Read the model definition and answer for the solid it produces. Units are mm, in the model's axes. A direction names the side the tool comes from. Coordinates: 2 decimals unless noted, no trailing zeros. Write each loop counter-clockwise with the first axis right and the second up, starting at its lowest first coordinate (ties: lowest second). Pieces come first, ordered by that corner, then holes.
1) The part is cut by section A-A (y = 23.5). Determine the outline of the cut face in (x, z), then the cut area to 3 significant figures.
2) Which of the six approach directions +Z, -Z, +X, -X, +Y, -Y give full straight-line access (tool end or side, diameter ignored) to faces 1 (the face through (84, 5, -2)), 2 (the face through (44, 17, 1)), 3 (the face through (64, 9.5, -70)), 4 (the face through (25.29, 5.19, -69.73)), 5 (the face through (44, 17, -94))?
3) The part is cut by section C-C (z = -78). Determine the outline of the cut face in (x, y).
4) The part is cut by section B-B (x = 14.85). Determine the outline of the cut face in (y, z).
5) Determine the mould class of faces 6 (the face through (73.06, 5.19, -87.65)), 7 (the face through (86, 5, -4)), 8 (the face through (44.126, 34.03, -91.986)) for opening direction X: +X half, -X half, draft (parallel to the pull), parting line (faces both ways), or undercut.
6) The part is cut by section D-D (x = 45). Determine the outline of the cut face in (y, z), then the cut area to 3 significant figures.
7) Each of these flat-tipped pins is pushed along its axis until it touches: pin 1 Ø0.6 at (x, y) = (85.5, 7) entering from -Z; pin 2 Ø3.5 at (x, z) = (5, -69) entering from +Y; pin 3 Ø2 at (y, z) = (4, -4) entering from -X. Where does it stop, or does it pass through?
8) Find the intervals of material crossed by line 1 (Z direction, x = 14.85, y = 0.4); line 2 (Z direction, x = 45, y = 19); line 3 (Y direction, x = 76, z = -38), in increasing order.
Autodesk Inventor part; units mm, degrees
ref_plane "YZ Plane" through (0, 0, 0) normal (1, 0, 0) x (0, 1, 0)
ref_plane "XZ Plane" through (0, 0, 0) normal (0, 1, 0) x (-1, 0, 0)
ref_plane "XY Plane" through (0, 0, 0) normal (0, 0, 1) x (1, 0, 0)
sketch "Sketch1" plane through (0, 0, 0) normal (0, 1, 0) x (-1, 0, 0)
  line L0 (0, 0) -> (-88, 0)
  line L1 (-88, 0) -> (-88, -94)
  line L2 (-88, -94) -> (0, -94)
  line L3 (0, -94) -> (0, 0)
  line L4 (0, -94) -> (0, -75.65)
  line L5 (0, -94) -> (-14.85, -94)
  circle A0 centre (-14.85, -75.65) radius 8.5
  line L6 (-44, -88.9444) -> (-44, -54.2543) construction
  circle A1 centre (-73.15, -75.65) radius 8.5
  dimension "d0" = 88
  dimension "d1" = 94
  dimension "d2" = 18.35
  dimension "d3" = 14.85
  dimension "d4" = 17
extrude "Extrusion1" add sketch "Sketch1" along normal blind 1
sketch "Sketch2" plane through (0, 1, 0) normal (0, 1, 0) x (1, 0, 0)
  line L0 (88, 94) -> (0, 94) construction
  line L1 (0, 94) -> (0, 0) construction
  line L2 (0, 0) -> (88, 0) construction
  line L3 (88, 0) -> (88, 94) construction
  circle A0 centre (73.15, 75.65) radius 8.5 construction
  circle A1 centre (14.85, 75.65) radius 8.5 construction
  line L4 (0, 94) -> (88, 94) construction
  line L5 (88, 94) -> (88, 95) construction
  line L6 (88, 95) -> (0, 95) construction
  line L7 (0, 95) -> (0, 94) construction
  line L8 (0, 0) -> (88, 0) construction
  line L9 (88, 0) -> (88, -1) construction
  line L10 (88, -1) -> (0, -1) construction
  line L11 (0, -1) -> (0, 0) construction
  line L12 (88, 95) -> (0, 95)
  line L13 (0, 95) -> (0, 94)
  line L14 (0, 94) -> (88, 94)
  line L15 (88, 94) -> (88, 95)
  line L16 (0, 0) -> (88, 0)
  line L17 (88, 0) -> (88, -1)
  line L18 (88, -1) -> (0, -1)
  line L19 (0, -1) -> (0, 0)
  dimension "d7" = 1
  dimension "d8" = 1
extrude "Extrusion2" add sketch "Sketch2" against normal blind 1
sketch "Sketch3" plane through (0, 1, 0) normal (0, 1, 0) x (1, 0, 0)
  line L0 (0, 95) -> (0, -1) construction
  line L1 (0, -1) -> (88, -1) construction
  line L2 (88, -1) -> (88, 95) construction
  line L3 (88, 95) -> (0, 95) construction
  circle A0 centre (73.15, 75.65) radius 8.5 construction
  circle A1 centre (14.85, 75.65) radius 8.5 construction
  line L4 (0, 0) -> (4, 0) construction
  line L5 (4, 0) -> (4, 4) construction
  line L6 (4, 4) -> (0, 4) construction
  line L7 (0, 4) -> (0, 0) construction
  line L8 (88, 0) -> (84, 0) construction
  line L9 (84, 0) -> (84, 4) construction
  line L10 (84, 4) -> (88, 4) construction
  line L11 (88, 4) -> (88, 0) construction
  line L12 (4, 4) -> (2, 4) construction
  line L13 (2, 4) -> (2, 2) construction
  line L14 (2, 2) -> (4, 2) construction
  line L15 (4, 2) -> (4, 4) construction
  line L16 (2, 2) -> (6, 2)
  line L17 (6, 2) -> (6, 4)
  line L18 (6, 4) -> (2, 4)
  line L19 (2, 4) -> (2, 2)
  line L20 (2, 2) -> (4, 2)
  line L21 (4, 2) -> (4, 6)
  line L22 (4, 6) -> (2, 6)
  line L23 (2, 6) -> (2, 2)
  line L24 (86, 2) -> (82, 2)
  line L25 (82, 2) -> (82, 4)
  line L26 (82, 4) -> (86, 4)
  line L27 (86, 4) -> (86, 2)
  line L28 (86, 2) -> (84, 2)
  line L29 (84, 2) -> (84, 6)
  line L30 (84, 6) -> (86, 6)
  line L31 (86, 6) -> (86, 2)
  line L32 (44, 4.3599) -> (37, 4.3599) construction
  line L33 (88, -1) -> (0, -1) construction
  line L34 (37, -1) -> (51, -1) construction
  line L35 (51, -1) -> (51, 0) construction
  line L36 (51, 0) -> (37, 0) construction
  line L37 (37, 0) -> (37, -1) construction
  line L38 (37, -1) -> (51, -1)
  line L39 (51, -1) -> (51, 0)
  line L40 (51, 0) -> (37, 0)
  line L41 (37, 0) -> (37, -1)
  line L42 (0, 95) -> (88, 95)
  line L43 (37, 95) -> (51, 95)
  line L44 (51, 95) -> (51, 94)
  line L45 (51, 94) -> (37, 94)
  line L46 (37, 94) -> (37, 95)
  circle A2 centre (14.85, 75.65) radius 10.5
  circle A3 centre (14.85, 75.65) radius 12
  line L47 (14.85, 75.65) -> (26.85, 75.65) construction
  line L48 (14.85, 75.65) -> (20.85, 86.0423) construction
  line L49 (14.85, 75.65) -> (8.85, 86.0423) construction
  line L50 (14.85, 75.65) -> (2.85, 75.65) construction
  line L51 (14.85, 75.65) -> (8.85, 65.2577) construction
  line L52 (14.85, 75.65) -> (20.85, 65.2577) construction
  line L53 (9.6, 84.7433) -> (8.85, 86.0423) construction
  line L54 (9.6, 84.7433) -> (8.85, 86.0423)
  line L55 (20.85, 86.0423) -> (20.1, 84.7433)
  line L56 (25.35, 75.65) -> (26.85, 75.65)
  line L57 (20.85, 65.2577) -> (20.1, 66.5567)
  line L58 (9.6, 66.5567) -> (8.85, 65.2577)
  line L59 (4.35, 75.65) -> (2.85, 75.65)
  line L60 (44, 84.7433) -> (44, 74.6259) construction
  circle A4 centre (73.15, 75.65) radius 8.5 construction
  circle A5 centre (73.15, 75.65) radius 10.5
  circle A6 centre (73.15, 75.65) radius 12
  line L61 (73.15, 75.65) -> (61.15, 75.65) construction
  line L62 (73.15, 75.65) -> (67.15, 86.0423) construction
  line L63 (73.15, 75.65) -> (79.15, 86.0423) construction
  line L64 (73.15, 75.65) -> (85.15, 75.65) construction
  line L65 (73.15, 75.65) -> (79.15, 65.2577) construction
  line L66 (73.15, 75.65) -> (67.15, 65.2577) construction
  line L67 (78.4, 84.7433) -> (79.15, 86.0423) construction
  line L68 (78.4, 84.7433) -> (79.15, 86.0423)
  line L69 (67.15, 86.0423) -> (67.9, 84.7433)
  line L70 (62.65, 75.65) -> (61.15, 75.65)
  line L71 (67.15, 65.2577) -> (67.9, 66.5567)
  line L72 (78.4, 66.5567) -> (79.15, 65.2577)
  line L73 (83.65, 75.65) -> (85.15, 75.65)
  point P0 (84, 4)
  dimension "d11" = 4
  dimension "d12" = 4
  dimension "d13" = 4
  dimension "d14" = 4
  dimension "d15" = 2
  dimension "d16" = 2
  dimension "d17" = 4
  dimension "d18" = 4
  dimension "d19" = 4
  dimension "d20" = 2
  dimension "d21" = 4
  dimension "d22" = 7
  dimension "d23" = 14
  dimension "d24" = 14
  dimension "d25" = 1
  dimension "d26" = 2
  dimension "d27" = 1.5
  dimension "d30" = 360
extrude "Extrusion3" add sketch "Sketch3" along normal blind 8.5 contours L19 L18 L21 L16 | L21 L18 L17 L16 | L23 L22 L21 L18 | L24 L29 L26 L27 | L24 L25 L26 L29 | L26 L29 L30 L31 | L56 A3 L57 A2 | A2 L54 A3 L55 | L58 A3 L59 A2 | L73 A6 L72 A5 | A5 L69 A6 L68 | L71 A6 L70 A5
sketch "Sketch4" plane through (0, 1, 0) normal (0, 1, 0) x (1, 0, 0)
  line L0 (2.85, 75.65) -> (4.35, 75.65) construction
  arc A0 (4.35, 75.65) -> (9.6, 66.5567) centre (14.85, 75.65) ccw construction
  line L1 (9.6, 66.5567) -> (8.85, 65.2577) construction
  arc A1 (2.85, 75.65) -> (8.85, 65.2577) centre (14.85, 75.65) ccw construction
  line L2 (84, 6) -> (86, 6) construction
  line L3 (86, 6) -> (86, 2) construction
  line L4 (86, 2) -> (82, 2) construction
  line L5 (82, 2) -> (82, 4) construction
  line L6 (82, 4) -> (84, 4) construction
  line L7 (84, 4) -> (84, 6) construction
  arc A2 (62.65, 75.65) -> (67.9, 66.5567) centre (73.15, 75.65) ccw construction
  line L8 (67.9, 66.5567) -> (67.15, 65.2577) construction
  arc A3 (61.15, 75.65) -> (67.15, 65.2577) centre (73.15, 75.65) ccw construction
  line L9 (61.15, 75.65) -> (62.65, 75.65) construction
  line L10 (25.35, 75.65) -> (26.85, 75.65) construction
  arc A4 (20.85, 65.2577) -> (26.85, 75.65) centre (14.85, 75.65) ccw construction
  line L11 (20.85, 65.2577) -> (20.1, 66.5567) construction
  arc A5 (20.1, 66.5567) -> (25.35, 75.65) centre (14.85, 75.65) ccw construction
  arc A6 (78.4, 84.7433) -> (67.9, 84.7433) centre (73.15, 75.65) ccw construction
  line L12 (67.9, 84.7433) -> (67.15, 86.0423) construction
  arc A7 (79.15, 86.0423) -> (67.15, 86.0423) centre (73.15, 75.65) ccw construction
  line L13 (79.15, 86.0423) -> (78.4, 84.7433) construction
  line L14 (2, 6) -> (4, 6) construction
  line L15 (4, 6) -> (4, 4) construction
  line L16 (4, 4) -> (6, 4) construction
  line L17 (6, 4) -> (6, 2) construction
  line L18 (6, 2) -> (2, 2) construction
  line L19 (2, 2) -> (2, 6) construction
  line L20 (83.65, 75.65) -> (85.15, 75.65) construction
  arc A8 (79.15, 65.2577) -> (85.15, 75.65) centre (73.15, 75.65) ccw construction
  line L21 (79.15, 65.2577) -> (78.4, 66.5567) construction
  arc A9 (78.4, 66.5567) -> (83.65, 75.65) centre (73.15, 75.65) ccw construction
  line L22 (20.85, 86.0423) -> (20.1, 84.7433) construction
  arc A10 (20.1, 84.7433) -> (9.6, 84.7433) centre (14.85, 75.65) ccw construction
  line L23 (9.6, 84.7433) -> (8.85, 86.0423) construction
  arc A11 (20.85, 86.0423) -> (8.85, 86.0423) centre (14.85, 75.65) ccw construction
  line L24 (0, 95) -> (0, -1) construction
  line L25 (0, -1) -> (88, -1) construction
  line L26 (88, -1) -> (88, 95) construction
  line L27 (88, 95) -> (0, 95) construction
  circle A12 centre (73.15, 75.65) radius 8.5 construction
  circle A13 centre (14.85, 75.65) radius 8.5 construction
  line L28 (44, 63.0064) -> (44, 95) construction
  line L29 (88, 95) -> (0, 95) construction
  line L30 (44, 95) -> (53, 95) construction
  line L31 (53, 95) -> (35, 95) construction
  line L32 (35, 95) -> (53, 95) construction
  line L33 (53, 95) -> (53, 94) construction
  line L34 (53, 94) -> (35, 94) construction
  line L35 (35, 94) -> (35, 95) construction
  line L36 (35, 95) -> (53, 95)
  line L37 (53, 95) -> (53, 94)
  line L38 (53, 94) -> (35, 94)
  line L39 (35, 94) -> (35, 95)
  line L40 (34.0602, 47) -> (52.5165, 47)
  line L41 (44, -1) -> (53, -1) construction
  line L42 (53, -1) -> (35, -1) construction
  line L43 (35, -1) -> (53, -1) construction
  line L44 (53, -1) -> (53, 0) construction
  line L45 (53, 0) -> (35, 0) construction
  line L46 (35, 0) -> (35, -1) construction
  line L47 (35, -1) -> (53, -1)
  line L48 (53, -1) -> (53, 0)
  line L49 (53, 0) -> (35, 0)
  line L50 (35, 0) -> (35, -1)
  point P0 (0, 0)
  dimension "d34" = 9
  dimension "d35" = 18
  dimension "d36" = 1
extrude "Extrusion4" add sketch "Sketch4" along normal blind 34.5
sketch "Sketch5" plane through (53, 1, 1) normal (1, 0, 0) x (0, 0, -1)
  line L0 (1, 0) -> (0, 0) construction
  line L1 (1, 0) -> (1, 34.5) construction
  line L2 (0, 34.5) -> (1, 34.5) construction
  line L3 (0, 0) -> (0, 34.5) construction
  line L4 (96, -1) -> (0, -1) construction
  line L5 (96, 0) -> (96, -1) construction
  line L6 (0, 0) -> (96, 0) construction
  line L7 (0, 0) -> (0, -1) construction
  line L8 (96, 0) -> (96, 34.5) construction
  line L9 (96, 0) -> (95, 0) construction
  line L10 (96, 0) -> (96, 34.5) construction
  line L11 (95, 34.5) -> (96, 34.5) construction
  line L12 (95, 0) -> (95, 34.5) construction
  line L13 (0, 34.5) -> (0, 31.6) construction
  line L14 (1, 31.6) -> (4, 31.6) construction
  line L15 (1, 34.5) -> (2, 34.5) construction
  line L16 (2, 34.5) -> (4, 31.6) construction
  line L17 (0, 34.5) -> (2, 34.5)
  line L18 (4, 31.6) -> (2, 34.5)
  line L19 (4, 31.6) -> (0, 31.6)
  line L20 (0, 31.6) -> (0, 34.5)
  line L21 (0, -1) -> (96, -1)
  line L22 (48, -1) -> (48, 2.5166)
  line L23 (95, 0) -> (95, 34.5) construction
  line L24 (96, 34.5) -> (95, 34.5) construction
  line L25 (96, 0) -> (96, 34.5) construction
  line L26 (96, 34.5) -> (96, 31.6) construction
  line L27 (95, 31.6) -> (92, 31.6) construction
  line L28 (95, 34.5) -> (94, 34.5) construction
  line L29 (94, 34.5) -> (92, 31.6) construction
  line L30 (96, 34.5) -> (94, 34.5)
  line L31 (92, 31.6) -> (94, 34.5)
  line L32 (92, 31.6) -> (96, 31.6)
  line L33 (96, 31.6) -> (96, 34.5)
  point P0 (1, -1)
  dimension "d39" = 2.9
  dimension "d40" = 3
  dimension "d41" = 1
extrude "Extrusion5" add sketch "Sketch5" against normal up to surface (18 mm away)
equation "\"d42\" = d40"
properties part number "case_v1"
Reported:
1. outline: (35, -95) - (53, -95) - (53, -94) - (35, -94) - close; (35, 0) - (53, 0) - (53, 1) - (35, 1) - close
1. area: 36.0 mm2
2. face 1: +Z, +X, -X, +Y
2. face 2: +Z, +X, -X, +Y, -Y
2. face 3: +Z, -Z, +X, -X, +Y
2. face 4: +Z, +Y
2. face 5: +X, -X
3. outline: (0, 0) - (6.68, 0) - (6.68, 1) - (0, 1) - close; (23.02, 0) - (64.98, 0) - (64.98, 1) - (23.02, 1) - close; (81.32, 0) - (88, 0) - (88, 1) - (81.32, 1) - close
4. outline: (0, -95) - (1, -95) - (1, -87.65) - (9.5, -87.65) - (9.5, -86.15) - (1, -86.15) - (1, -84.15) - (0, -84.15) - close; (0, -67.15) - (1, -67.15) - (1, 1) - (0, 1) - close
5. face 6: undercut
5. face 7: +X half
5. face 8: draft
6. outline: (0, -95) - (35.5, -95) - (35.5, -93) - (32.6, -91) - (32.6, -94) - (1, -94) - (1, 0) - (32.6, 0) - (32.6, -3) - (35.5, -1) - (35.5, 1) - (0, 1) - close
6. area: 177 mm2
7. pin 1: stops at z = -6
7. pin 2: stops at y = 9.5
7. pin 3: stops at x = 2
8. line 1: z = -95 to -84.15, -67.15 to 1
8. line 2: z = -95 to -94, 0 to 1
8. line 3: y = 0 to 1
